Geometry: final body of the model. Coordinates: model frame, mm. Round coordinates to 2 decimals unless told otherwise and drop trailing zeros. Write each loop counter-clockwise with the first axis right and the second up, starting at its lowest first coordinate (ties: lowest second). Pieces come first, ordered by that corner, then holes.
from build123d import *

# Parameters (mm, degrees)
SKETCH1_W                     = 25.4
SKETCH1_H                     = 98.425
SKETCH1_W_2                   = 203.2
SKETCH1_H_2                   = 19.05
BOSS_EXTRUDE1_DEPTH           = 1.5875
FILLET2_R                     = 3.175
TAP_DRILL_FOR_1_4_HELICOIL0_D = 6.7564


with BuildPart() as part:
    # Sketch1 → Boss-Extrude1 (new body)
    with BuildSketch(Plane(origin=(0, 0, 0), x_dir=(1, 0, 0), z_dir=(0, 1, 0))):
        with Locations((-114.3, 0)):
            Rectangle(SKETCH1_W, SKETCH1_H)
        with Locations((0, -39.6875)):
            Rectangle(SKETCH1_W_2, SKETCH1_H_2)
        Polygon((101.6, 49.2125), (101.6, -30.1625), (101.6, -49.2125), (127, -49.2125), (127, 49.2125), align=None)
    extrude(amount=BOSS_EXTRUDE1_DEPTH)

    # Fillet2
    fillet2_edges = [part.edges().sort_by_distance(p)[0] for p in [
        (-101.6, 0.79375, 30.1625),
        (101.6, 0.79375, 30.1625),
        (101.6, 0.79375, -49.2125),
        (127, 0.79375, -49.2125),
        (127, 0.79375, 49.2125),
        (-127, 0.79375, 49.2125),
        (-127, 0.79375, -49.2125),
        (-101.6, 0.79375, -49.2125),
    ]]
    fillet(fillet2_edges, radius=FILLET2_R)

    # Tap Drill for 1/4 Helicoil0 (through all)
    with Locations(Plane(origin=(0, 1.5875, 0), x_dir=(1, 0, 0), z_dir=(0, 1, 0))):
        with Locations((-114.3, 36.5125), (-114.3, 11.1125), (-114.3, -14.2875), (-57.15, -39.6875), (0, -39.6875), (57.15, -39.6875), (114.3, -14.2875), (114.3, 11.1125), (114.3, 36.5125), (-114.3, -39.6875), (114.3, -39.6875)):
            Hole(TAP_DRILL_FOR_1_4_HELICOIL0_D / 2)


solid = part.part
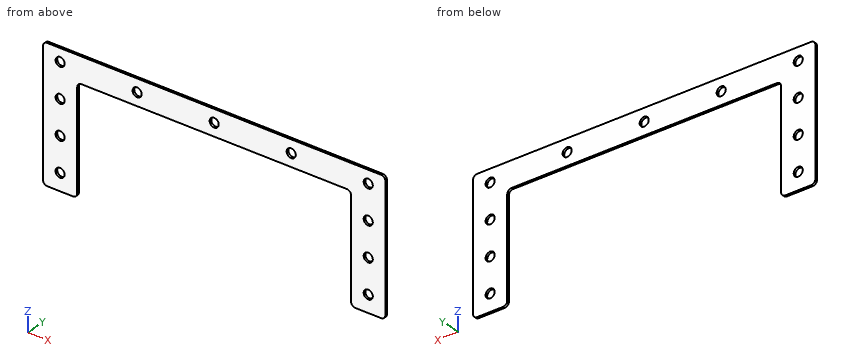
1) Section A-A on z = 3.5. Output: boundary loops of the cut face in (x, y).
2) Section C-C on x = -114.3. Output: boundary loops of the cut face in (y, z), plus the area to 3 significant figures.
3) First-contact query: P1, Ø4, axis at x = 0, z = 39.69, coming from the +Y side; P2, Ø0.5, axis at x = 6, y = 0.5, coming from the -Z side. Flat tips, straight axial feed; report the tip coordinate or a pass-through.
4) Section B-B on x = -57.15. Output: boundary loops of the cut face in (y, z), plus the area to 3 significant figures.
5) Section D-D on y = 1.2. State how many separate pieces and enclosed holes the cut face has, plus the area to 3 significant figures.
6) Line query: probe 1 along Z at (x, y) = (-114.3, 0.45); probe 2 along X at (y, z) = (0.5, 27.5); probe 3 along X at (y, z) = (0.15, 12.5). Output: solid intervals per line, ascending.
Filled in:
1. outline: (-127, 0) - (-101.6, 0) - (-101.6, 1.59) - (-127, 1.59) - close; (101.6, 0) - (127, 0) - (127, 1.59) - (101.6, 1.59) - close
2. outline: (0, -49.21) - (1.59, -49.21) - (1.59, -39.89) - (0, -39.89) - close; (0, -33.13) - (1.59, -33.13) - (1.59, -14.49) - (0, -14.49) - close; (0, -7.73) - (1.59, -7.73) - (1.59, 10.91) - (0, 10.91) - close; (0, 17.67) - (1.59, 17.67) - (1.59, 36.31) - (0, 36.31) - close; (0, 43.07) - (1.59, 43.07) - (1.59, 49.21) - (0, 49.21) - close
2. area: 113 mm2
3. P1: passes through
3. P2: stops at z = 30.16
4. outline: (0, 30.16) - (1.59, 30.16) - (1.59, 36.31) - (0, 36.31) - close; (0, 43.07) - (1.59, 43.07) - (1.59, 49.21) - (0, 49.21) - close
4. area: 19.5 mm2
5. separate pieces: 1
5. enclosed holes: 11
5. area: 8,470 mm2
6. probe 1: z = -49.21 to -39.89, -33.13 to -14.49, -7.73 to 10.91, 17.67 to 36.31, 43.07 to 49.21
6. probe 2: x = -127 to -101.56, 101.56 to 127
6. probe 3: x = -127 to -117.17, -111.43 to -101.6, 101.6 to 111.43, 117.17 to 127
